from build123d import *

# Parameters (mm, degrees)
SKETCH1_W           = 140
SKETCH1_H           = 154
SKETCH1_R           = 6.5
BOSS_EXTRUDE1_DEPTH = 6


with BuildPart() as part:
    # Sketch1 → Boss-Extrude1 (new body, symmetric)
    with BuildSketch(Plane.XY):
        Rectangle(SKETCH1_W, SKETCH1_H)
        with Locations((-54, 61)):
            Circle(SKETCH1_R, mode=Mode.SUBTRACT)
        with Locations((54, 61)):
            Circle(SKETCH1_R, mode=Mode.SUBTRACT)
        with Locations((-54, -61)):
            Circle(SKETCH1_R, mode=Mode.SUBTRACT)
        with Locations((54, -61)):
            Circle(SKETCH1_R, mode=Mode.SUBTRACT)
    extrude(amount=BOSS_EXTRUDE1_DEPTH, both=True)


solid = part.part
The listing builds one solid part. Answer for the finished solid, in the listing's coordinates (mm). Round coordinates to 2 decimals unless told otherwise and drop trailing zeros. Write each loop counter-clockwise with the first axis right and the second up, starting at its lowest first coordinate (ties: lowest second). Pieces come first, ordered by that corner, then holes. Notation, with made-up numbers: (74, 22) - (82, 22) arc R22 cw to (82, 38) - close; hole circle Ø8 at (73, -20). An arc over 180 degrees is marked (long way). Use a Markdown table: item, result. Add a question column.
1. The part is cut by section C-C (z = 1). Write down the section's boundary in (x, y).
2. Consider line 1 (Y direction, x = 54, z = 2.5); line 2 (X direction, y = -63, z = 5); line 3 (Y direction, x = -50, z = 2.5). Determine where each line is inside the solid, lowest interval first.
3. The part is cut by section A-A (y = 61). Write down the section's boundary in (x, z).
4. The part is cut by section B-B (x = -54). Write down the section's boundary in (y, z), and give its area (3 significant figures).
5. Flat-ended cylindrical pins translate along their axes: P1, Ø21, axis at x = 54, y = -61, coming from the +Z side; P2, Ø8, axis at x = -54, y = -61, coming from the -Z side. Find the tip coordinate at first contact, or state that the pin passes through.
6. For a pull along X with two mould halves and no side action, classify faces 1 (the face through (70, -1, 0)), 2 (the face through (-1, 77, 0)), 3 (the face through (-55.409, -67.345, -0.084)) as +X half, -X half, draft (parallel to the pull), parting line (faces both ways), or undercut.
Reported:
| question | item | result |
|---|---|---|
| 1 | outline | (-70, -77) - (70, -77) - (70, 77) - (-70, 77) - close; hole circle Ø13 at (-54, -61); hole circle Ø13 at (-54, 61); hole circle Ø13 at (54, -61); hole circle Ø13 at (54, 61) |
| 2 | line 1 | -77 to -67.5, -54.5 to 54.5, 67.5 to 77 |
| 2 | line 2 | -70 to -60.18, -47.82 to 47.82, 60.18 to 70 |
| 2 | line 3 | -77 to -66.12, -55.88 to 55.88, 66.12 to 77 |
| 3 | outline | (-70, -6) - (-60.5, -6) - (-60.5, 6) - (-70, 6) - close; (-47.5, -6) - (47.5, -6) - (47.5, 6) - (-47.5, 6) - close; (60.5, -6) - (70, -6) - (70, 6) - (60.5, 6) - close |
| 4 | outline | (-77, -6) - (-67.5, -6) - (-67.5, 6) - (-77, 6) - close; (-54.5, -6) - (54.5, -6) - (54.5, 6) - (-54.5, 6) - close; (67.5, -6) - (77, -6) - (77, 6) - (67.5, 6) - close |
| 4 | area | 1,540 mm^2 |
| 5 | P1 | z = 6 |
| 5 | P2 | through |
| 6 | face 1 | +X half |
| 6 | face 2 | draft |
| 6 | face 3 | undercut |
